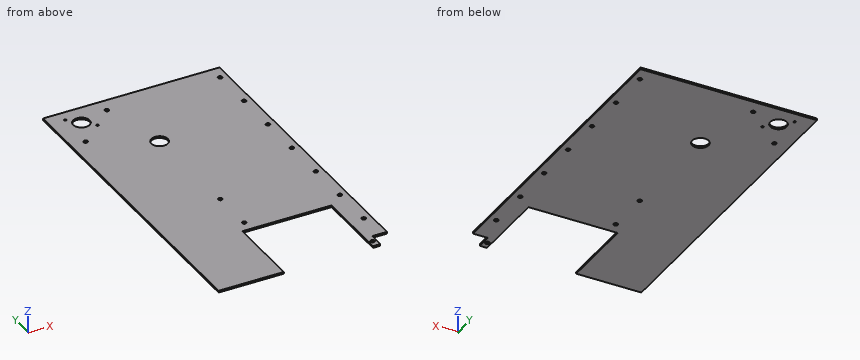
Autodesk Inventor part; units mm, degrees
ref_plane "YZ Plane" through (0, 0, 0) normal (1, 0, 0) x (0, 1, 0)
ref_plane "XZ Plane" through (0, 0, 0) normal (0, 1, 0) x (-1, 0, 0)
ref_plane "XY Plane" through (0, 0, 0) normal (0, 0, 1) x (1, 0, 0)
sketch "Sketch1" plane through (0, 0, 0) normal (0, 0, 1) x (1, 0, 0)
  line L0 (-115.6368, 165.4342) -> (189.1632, 165.4342)
  line L1 (189.1632, 165.4342) -> (189.1632, -393.3658)
  line L2 (189.1632, -393.3658) -> (-115.6368, -393.3658)
  line L3 (-115.6368, -393.3658) -> (-115.6368, 165.4342)
  line L4 (151.0632, -393.3658) -> (151.0632, -261.2858)
  line L5 (189.1632, -393.3658) -> (163.5092, -393.3658)
  line L6 (163.5092, -393.3658) -> (163.5092, -367.7118)
  line L7 (163.5092, -367.7118) -> (189.1632, -367.7118)
  line L8 (189.1632, -367.7118) -> (189.1632, -393.3658)
  line L9 (151.0632, -261.2858) -> (-3.064, -261.2858)
  line L10 (-3.064, -261.2858) -> (-3.064, -393.3658)
  circle A0 centre (157.2862, -380.5388) radius 3.5687
  line L11 (189.1632, -317.1658) -> (-115.6368, -317.1658)
  circle A1 centre (9.0264, 24.007) radius 14.2875
  point P0 (0, 0)
  dimension "d0" = 304.8
  dimension "d1" = 558.8
  dimension "d2" = 180.1368
  dimension "d3" = 417.3728
  dimension "d4" = 38.1
  dimension "d5" = 25.654
  dimension "d6" = 25.654
  dimension "d7" = 154.1272
  dimension "d10" = 132.08
  dimension "d11" = 12.446
  dimension "d12" = 6.223
  dimension "d13" = 12.827
  dimension "d14" = 7.1374
  dimension "d15" = 76.2
  dimension "d16" = 28.575
extrude "Extrusion1" add sketch "Sketch1" along normal blind 3.175 contours L0 L1 L11 L4 L9 L10 L3 | L11 L10 L2 L3 | L1 L7 L6 L2 L4 L11
sketch "Sketch2" plane through (0, 0, 3.175) normal (0, 0, 1) x (1, 0, 0)
  line L0 (151.0632, -393.3658) -> (163.5092, -393.3658)
  line L1 (189.1632, -367.7118) -> (189.1632, 165.4342)
  point P0 (0, 0)
  point P1 (176.4632, -317.1658)
  point P2 (176.4632, -240.9658)
  point P3 (176.4632, -164.7658)
  point P4 (176.4632, -88.5658)
  point P5 (176.4632, -12.3658)
  point P6 (176.4632, 63.8342)
  point P7 (176.4632, 140.0342)
  point P8 (11.3632, -240.9658)
  point P9 (11.3632, -164.7658)
  dimension "d20" = 76.2
  dimension "d21" = 12.7
  dimension "d22" = 76.2
  dimension "d23" = 76.2
  dimension "d24" = 76.2
  dimension "d25" = 76.2
  dimension "d26" = 76.2
  dimension "d27" = 76.2
  dimension "d29" = 165.1
  dimension "d30" = 165.1
hole "Hole1" at (176.4632, -317.1658, 3.175) at (176.4632, -240.9658, 3.175) at (176.4632, -164.7658, 3.175) at (176.4632, -88.5658, 3.175) at (176.4632, -12.3658, 3.175) at (176.4632, 63.8342, 3.175) at (176.4632, 140.0342, 3.175) at (11.3632, -240.9658, 3.175) at (11.3632, -164.7658, 3.175) direction (0, 0, -1) diameter 7.1374 end through all
sketch "Sketch4" plane through (0, 0, 3.175) normal (0, 0, 1) x (1, 0, 0)
  circle A0 centre (-69.9042, 127.3342) radius 14.195
  circle A1 centre (-87.8647, 145.2947) radius 2.0193
  circle A2 centre (-51.9436, 109.3737) radius 2.0193
  line L0 (-90.9042, 134.5342) -> (-90.9042, 120.1342)
  line L1 (-90.9042, 120.1342) -> (-92.1292, 118.9092)
  line L2 (-92.1292, 118.9092) -> (-92.1292, 113.3342)
  line L3 (-92.1292, 113.3342) -> (-85.9042, 113.3342)
  arc A3 (-83.9042, 111.3342) -> (-85.9042, 113.3342) centre (-85.9042, 111.3342) ccw
  line L4 (-83.9042, 111.3342) -> (-83.9042, 106.3342)
  line L5 (-83.9042, 106.3342) -> (-49.9042, 106.3342)
  arc A4 (-49.9042, 106.3342) -> (-48.9042, 107.3342) centre (-69.9042, 127.3342) ccw
  line L6 (-48.9042, 107.3342) -> (-48.9042, 109.1342)
  line L7 (-48.9042, 109.1342) -> (-47.6792, 110.3592)
  line L8 (-47.6792, 110.3592) -> (-47.6792, 118.9092)
  line L9 (-47.6792, 118.9092) -> (-48.9042, 120.1342)
  line L10 (-48.9042, 120.1342) -> (-48.9042, 134.5342)
  line L11 (-48.9042, 134.5342) -> (-47.6792, 135.7592)
  line L12 (-47.6792, 135.7592) -> (-47.6792, 141.3342)
  line L13 (-47.6792, 141.3342) -> (-53.9042, 141.3342)
  arc A5 (-55.9042, 143.3342) -> (-53.9042, 141.3342) centre (-53.9042, 143.3342) ccw
  line L14 (-55.9042, 143.3342) -> (-55.9042, 148.3342)
  line L15 (-55.9042, 148.3342) -> (-89.9042, 148.3342)
  arc A6 (-89.9042, 148.3342) -> (-90.9042, 147.3342) centre (-69.9042, 127.3342) ccw
  line L16 (-90.9042, 147.3342) -> (-90.9042, 145.5342)
  line L17 (-90.9042, 145.5342) -> (-92.1292, 144.3092)
  line L18 (-92.1292, 144.3092) -> (-92.1292, 135.7592)
  line L19 (-92.1292, 135.7592) -> (-90.9042, 134.5342)
  circle A7 centre (9.0264, 24.007) radius 14.2875
  line L20 (189.1632, 165.4342) -> (-115.6368, 165.4342)
  line L21 (-115.6368, 165.4342) -> (-115.6368, -393.3658)
  point P0 (0, 0)
  dimension "d50" = 3.0395
  dimension "d51" = 4.2645
  dimension "d52" = 4.2645
  dimension "d53" = 3.0395
  dimension "d54" = 130.0251
  dimension "d55" = 21
  dimension "d56" = 21
  dimension "d57" = 38.1
  dimension "d59" = 45.7327
extrude "Extrusion3" cut sketch "Sketch4" against normal blind 25.4 contours A0 | A1 | A2
sketch "Sketch5" plane through (0, 0, 3.175) normal (0, 0, 1) x (1, 0, 0)
  line L0 (-115.6368, 165.4342) -> (-115.6368, -393.3658)
  line L1 (189.1632, 165.4342) -> (-115.6368, 165.4342)
  circle A0 centre (-69.9042, 127.3342) radius 14.195
  point P0 (0, 0)
  point P1 (-90.2368, 76.5342)
  point P2 (-19.1042, 140.0342)
  dimension "d62" = 25.4
  dimension "d63" = 25.4
  dimension "d64" = 50.8
  dimension "d65" = 50.8
hole "Hole2" at (-90.2368, 76.5342, 3.175) at (-19.1042, 140.0342, 3.175) direction (0, 0, -1) diameter 7.1374 end through all
properties part number "GearboxPlateRev2"
Work out the finished part from the listing and answer in its coordinate system (mm). Coordinates: 2 decimals unless noted, no trailing zeros. Loops run counter-clockwise (first coordinate to the right, second up) from the corner with the lowest first, then second, coordinate; pieces in that order, holes last. Notation, with made-up numbers: M 43,3.5 L 73,3.5 A18 ccw 73,36.5 Z; hole C 19,42 d2. An arc over 180 degrees is marked long. Answer in a Markdown table with one row per item. Add a question column.
1. Consider L1, parallel to Y at x = 14.5, z = 0.4; L2, parallel to X at y = -303, z = 2.85; L3, parallel to Y at x = 13, z = 1.35. Determine where each line is inside the solid, lowest interval first.
2. Find section D-D, the plane y = 16.5. Write down the section's boundary in (x, z) (3 decimals), then the cut area to 3 significant figures.
3. Find section A-A, the plane y = -286. Write down the section's boundary in (x, z) (3 decimals).
4. Find section C-C, the plane x = 79.5. Write down the section's boundary in (y, z) (3 decimals).
5. Flat-ended cylindrical pins translate along their axes: P1, Ø17, axis at x = 9.03, y = 24.01, coming from the -Z side; P2, Ø1.6, axis at x = 176, z = 1.5, coming from the -Y side. Find the tip coordinate at first contact, or state that the pin passes through.
6. Find section B-B, the plane z = 0.5. State how many separate pieces and enclosed holes the cut face has, then the cut area to 3 significant figures.
Reported:
| question | item | result |
|---|---|---|
| 1 | L1 | y = -261.29 to -242.67, -239.26 to -166.47, -163.06 to 10.81, 37.2 to 165.43 |
| 1 | L2 | x = -115.64 to -3.06, 151.06 to 189.16 |
| 1 | L3 | y = -261.29 to -244.14, -237.79 to -167.94, -161.59 to 10.28, 37.73 to 165.43 |
| 2 | outline | M -115.637,0 L -3.13,0 L -3.13,3.175 L -115.637,3.175 Z; M 21.183,0 L 189.163,0 L 189.163,3.175 L 21.183,3.175 Z |
| 2 | area | 891 mm^2 |
| 3 | outline | M -115.637,0 L -3.064,0 L -3.064,3.175 L -115.637,3.175 Z; M 151.063,0 L 189.163,0 L 189.163,3.175 L 151.063,3.175 Z |
| 4 | outline | M -261.286,0 L 165.434,0 L 165.434,3.175 L -261.286,3.175 Z |
| 5 | P1 | passes through |
| 5 | P2 | stops at y = -367.71 |
| 6 | separate pieces | 1 |
| 6 | enclosed holes | 16 |
| 6 | area | 148,000 mm^2 |
